Design review of the part built by this model. Coordinates are the model's own, in mm. Face numbers are marked on the shaded views. A direction names the side the tool comes from. Give positions to 0.01 mm unless a question says otherwise; leave off trailing zeros. Write each loop counter-clockwise with the first axis right and the second up, starting at its lowest first coordinate (ties: lowest second). Pieces come first, ordered by that corner, then holes. Notation, with made-up numbers: (47, 74) -> (79, 74) arc R21 cw to (79, 105) -> close; hole circle Ø3 at (50, 29.25). An arc over 180 degrees is marked (long way). Write each question's results on one line, items separated by ' | '. Start each with the question number.
(1) For the marked faces 1, 2 and 3, list the 3-axis set-ups (+Z, -Z, +X, -X, +Y, -Y) from which the entire face can be reached by the end or side of a thin tool; tool diameter is ignored.
(2) To check wall thickness, follow probe 1 along Y at (x, z) = (0, -4.5); probe 2 along Y at (x, z) = (0, -15); probe 3 along Y at (x, z) = (12.5, -4.25). State the ranges of each line that lie inside material, in increasing order.
(3) Take a section at A-A (y = 0). State the section outline as (x, z) points.
(4) Mouldability with a two-part tool opening along Y and no side actions: class the marked faces 4, 5 and 6 as released by +Y, released by -Y, zero draft, split by the parting line, or undercut.
(5) Take a section at D-D (z = -2.5). State the section outline as (x, y) points, plus the area to 3 significant figures.
(6) Take a section at C-C (z = -13). State the section outline as (x, y) points.
(7) Clearance check with flat-ended pins moving along their axes: pin 1 (8.5 mm diameter, centred on x = 0, y = 0, fed in from -Z); pin 2 (10 mm diameter, centred on x = 9.5, z = -12.5, fed in from -Y); pin 3 (2 mm diameter, centred on x = 0, y = -12.5, fed in from +Z); pin 4 (10 mm diameter, centred on y = -9.5, z = -6, fed in from -X). State where each tip first meets the part, or that it passes through.
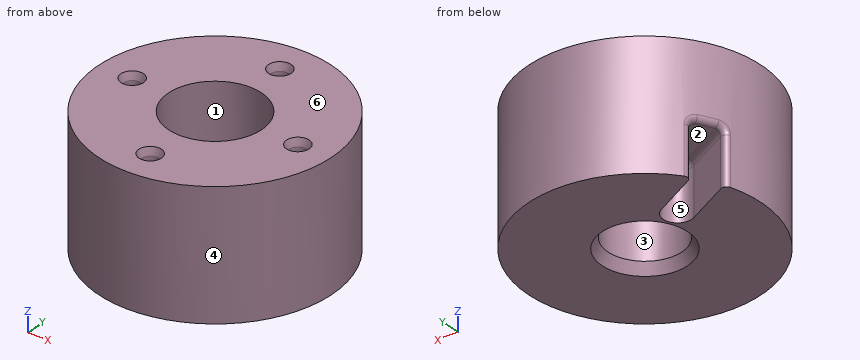
from build123d import *

# Parameters (mm, degrees)
SKETCH_1_R          = 17.5
EXTRUDE_1_DEPTH     = 19
SKETCH_2_R          = 1.3
CUT_EXTRUDE_1_DEPTH = 8
SKETCH_4_R          = 7
CUT_EXTRUDE_3_DEPTH = 9
SKETCH_5_R          = 5.55
CUT_EXTRUDE_4_DEPTH = 10
CUT_EXTRUDE_START   = -8
CUT_EXTRUDE_6_DEPTH = 8
FILLET_2_R          = 0.8
CHAMFER_1_SIZE      = 0.9
CHAMFER_1_SIZE2     = 1.558845727
CHAMFER_2_SIZE      = 0.4
CHAMFER_2_SIZE2     = 1.098990968
FILLET_3_R          = 0.8


with BuildPart() as part:
    # 草图1 → 凸台-拉伸1 (new body)
    with BuildSketch(Plane.XY):
        Circle(SKETCH_1_R)
    extrude(amount=-EXTRUDE_1_DEPTH)

    # 草图2 → 切除-拉伸1 (cut)
    with BuildSketch(Plane.XY):
        with Locations((12.5, 0)):
            Circle(SKETCH_2_R)
        with Locations((0, -12.5)):
            Circle(SKETCH_2_R)
        with Locations((-12.5, 0)):
            Circle(SKETCH_2_R)
        with Locations((0, 12.5)):
            Circle(SKETCH_2_R)
    extrude(amount=-CUT_EXTRUDE_1_DEPTH, mode=Mode.SUBTRACT)

    # 草图4 → 切除-拉伸3 (cut)
    with BuildSketch(Plane.XY):
        Circle(SKETCH_4_R)
    extrude(amount=-CUT_EXTRUDE_3_DEPTH, mode=Mode.SUBTRACT)

    # 草图5 → 切除-拉伸4 (cut)
    with BuildSketch(Plane.XY.offset(-9)):
        Circle(SKETCH_5_R)
    extrude(amount=-CUT_EXTRUDE_4_DEPTH, mode=Mode.SUBTRACT)

    # 草图6 → 切除-拉伸6 (cut)
    with BuildSketch(Plane(origin=(0, 0, -19), x_dir=(-1, 0, 0), z_dir=(0, 0, -1)).offset(CUT_EXTRUDE_START)):
        with BuildLine():
            Line((7.095083956, 5.939889195), (14.583381366, 9.673416559))
            ThreePointArc((14.583381366, 9.673416559), (15.661351328, 7.808461729), (16.502031962, 5.825198805))
            Line((16.502031962, 5.825198805), (9.013734553, 2.091671441))
            ThreePointArc((9.013734553, 2.091671441), (6.130300377, 3.05645502), (7.095083956, 5.939889195))
        make_face()
    extrude(amount=CUT_EXTRUDE_6_DEPTH, mode=Mode.SUBTRACT)

    # 圆角2
    fillet_2_edges = [part.edges().sort_by_distance(p)[0] for p in [
        (-6.130300377, 3.05645502, -11),
        (-10.839232661, 7.806652877, -11),
        (-12.757883257, 3.958435123, -11),
    ]]
    fillet(fillet_2_edges, radius=FILLET_2_R)

    # 倒角1
    chamfer_1_edges = [part.edges().sort_by_distance(p)[0] for p in [
        (-5.55, 0, -19),
    ]]
    chamfer_1_side = [part.faces().sort_by_distance(p)[0] for p in [
        (-2.871452094, -16.760836695, -19),
    ]]
    chamfer(chamfer_1_edges, length=CHAMFER_1_SIZE, length2=CHAMFER_1_SIZE2, reference=chamfer_1_side[0])

    # 倒角2
    chamfer_2_edges = [part.edges().sort_by_distance(p)[0] for p in [
        (-1.3, -12.5, 0),
        (-13.8, 0, 0),
        (-1.3, 12.5, 0),
        (11.2, 0, 0),
    ]]
    chamfer_2_side = [part.faces().sort_by_distance(p)[0] for p in [
        (-17.005025253, 0, 0),
    ]]
    chamfer(chamfer_2_edges, length=CHAMFER_2_SIZE, length2=CHAMFER_2_SIZE2, reference=chamfer_2_side[0])

    # 圆角3
    fillet_3_edges = [part.edges().sort_by_distance(p)[0] for p in [
        (-15.661351328, 7.808461729, -11),
        (-16.502031962, 5.825198805, -15.4),
        (-14.583381366, 9.673416559, -15.4),
        (-16.421826211, 6.047613073, -11.233795824),
        (-14.712740273, 9.475509151, -11.233795824),
    ]]
    fillet(fillet_3_edges, radius=FILLET_3_R)


solid = part.part
Report:
1) face 1: +Z | face 2: -Z | face 3: +Z, -Z
2) probe 1: -17.5 to -13.8, -11.2 to -7, 7 to 11.2, 13.8 to 17.5 | probe 2: -17.5 to -5.55, 5.55 to 17.5 | probe 3: -12.25 to -1.3, 1.3 to 12.25
3) outline: (-17.5, -19) -> (-6.45, -19) -> (-5.55, -17.44) -> (-5.55, -9) -> (-7, -9) -> (-7, 0) -> (-10.8, 0) -> (-11.2, -1.1) -> (-11.2, -8) -> (-13.8, -8) -> (-13.8, -1.1) -> (-14.2, 0) -> (-17.5, 0) -> close; (5.55, -17.44) -> (6.45, -19) -> (17.5, -19) -> (17.5, 0) -> (14.2, 0) -> (13.8, -1.1) -> (13.8, -8) -> (11.2, -8) -> (11.2, -1.1) -> (10.8, 0) -> (7, 0) -> (7, -9) -> (5.55, -9) -> close
4) face 4: split by the parting line | face 5: undercut | face 6: zero draft
5) outline: circle Ø35 at (0, 0); hole circle Ø2.6 at (-12.5, 0); hole circle Ø14 at (0, 0); hole circle Ø2.6 at (0, -12.5); hole circle Ø2.6 at (0, 12.5); hole circle Ø2.6 at (12.5, 0) | area: 787 mm2
6) outline: (-16.79, 4.92) arc R17.5 ccw (long way) to (-14.04, 10.45) arc R0.8 ccw to (-13.75, 9.26) -> (-7.1, 5.94) arc R2.15 cw to (-9.01, 2.09) -> (-15.67, 5.41) arc R0.8 ccw to start; hole circle Ø11.1 at (0, 0)
7) pin 1: through | pin 2: y = -16.91 | pin 3: z = -8 | pin 4: x = -16.91
